CAD build for the part. Positions are in the model's coordinates, mm. A direction names the side the tool comes from. Round coordinates to 2 decimals unless told otherwise and drop trailing zeros. Loops run counter-clockwise (first coordinate to the right, second up) from the corner with the lowest first, then second, coordinate; pieces in that order, holes last. Notation, with made-up numbers: M 35,57 L 79,57 A22 ccw 79,67 Z; hole C 59,-39 d1. An arc over 180 degrees is marked long. Use one line per item in the form item = value.
from build123d import *

# Parameters (mm, degrees)
F0_W     = 105.6
F0_H     = 29.4
F0_W_2   = 10
F0_H_2   = 80
F1_DEPTH = 4
F2_W     = 105.6
F2_H     = 29.4
F3_DEPTH = 1.5
F4_R     = 2


with BuildPart() as f1:
    # F0 (on Top) → F1 (new body)
    with BuildSketch(Plane.XY):
        Polygon((57.8, 19.7), (-57.8, 19.7), (-57.8, -19.7), (-5, -19.7), (5, -19.7), (57.8, -19.7), align=None)
        Rectangle(F0_W, F0_H, mode=Mode.SUBTRACT)
        Rectangle(F0_W, F0_H)
        with Locations((0, -59.7)):
            Rectangle(F0_W_2, F0_H_2)
        Polygon((5, -99.7), (-5, -99.7), (0, -121.124285), align=None)
    extrude(amount=F1_DEPTH)

    # F2 (on face) → F3 (cut)
    with BuildSketch(Plane.XY.offset(4)):
        Rectangle(F2_W, F2_H)
    extrude(amount=-F3_DEPTH, mode=Mode.SUBTRACT)

    # F4
    f4_edges = [f1.edges().sort_by_distance(p)[0] for p in [
        (-57.8, 19.7, 2),
        (-57.8, -19.7, 2),
        (57.8, -19.7, 2),
        (57.8, 19.7, 2),
        (52.8, 14.7, 3.25),
        (-52.8, 14.7, 3.25),
        (-52.8, -14.7, 3.25),
        (52.8, -14.7, 3.25),
        (5, -19.7, 2),
        (-5, -19.7, 2),
    ]]
    fillet(f4_edges, radius=F4_R)


solid = f1.part
1. Cut at A-A on y = -8.5. Write the cut outline in (x, z), and give its area (3 significant figures).
Completed:
outline = M -57.8,0 L 57.8,0 L 57.8,4 L 52.8,4 L 52.8,2.5 L -52.8,2.5 L -52.8,4 L -57.8,4 Z
area = 304 mm2
2. Cut at D-D on y = -94. Write the cut outline in (x, z), and give its area (3 significant figures).
Completed:
outline = M -5,0 L 5,0 L 5,4 L -5,4 Z
area = 40.0 mm2
3. Tool access for faces 1 (the face through (-1, 0, 2.5)), 2 (the face through (31, -19.7, 2)), 3 (the face through (-32, -19.7, 2)), 4 (the face through (-1, -18, 0)): list every direction of +Z, -Z, +X, -X, +Y, -Y with a clear straight run to the whole face (end or side of a thin tool).
Completed:
face_1 = +Z
face_2 = +Z, -Z, +X, -Y
face_3 = +Z, -Z, -X, -Y
face_4 = -Z, +X, -X, +Y, -Y
4. Cut at B-B on z = 1.75. Write the cut outline in (x, y), and give its area (3 significant figures).
Completed:
outline = M -57.8,-17.7 A2 ccw -55.8,-19.7 L -7,-19.7 A2 cw -5,-21.7 L -5,-99.7 L 0,-121.12 L 5,-99.7 L 5,-21.7 A2 cw 7,-19.7 L 55.8,-19.7 A2 ccw 57.8,-17.7 L 57.8,17.7 A2 ccw 55.8,19.7 L -55.8,19.7 A2 ccw -57.8,17.7 Z
area = 5,460 mm2
5. Cut at C-C on x = -38. Write the cut outline in (y, z).
Completed:
outline = M -19.7,0 L 19.7,0 L 19.7,4 L 14.7,4 L 14.7,2.5 L -14.7,2.5 L -14.7,4 L -19.7,4 Z
6. Drop flat-ended pins along their axis: P1, Ø2, axis at x = 3.5, y = -12, coming from the +Z side; P2, Ø1, axis at x = -36.5, z = 1.5, coming from the -Y side; P3, Ø2, axis at y = -61, z = 3.5, coming from the -X side. Give the stop position or say it passes through.
Completed:
P1 = 2.5
P2 = -19.7
P3 = -5
7. Probe line 1 along Y through (x, z) = (38.5, 3.8); line 2 along Z through (x, y) = (15.5, 10.5); line 3 along X through (y, z) = (-79, 2.1). List the from-to ranges inside material, lowest first. Write a range as from..to.
Completed:
line_1 = -19.7..-14.7, 14.7..19.7
line_2 = 0..2.5
line_3 = -5..5
